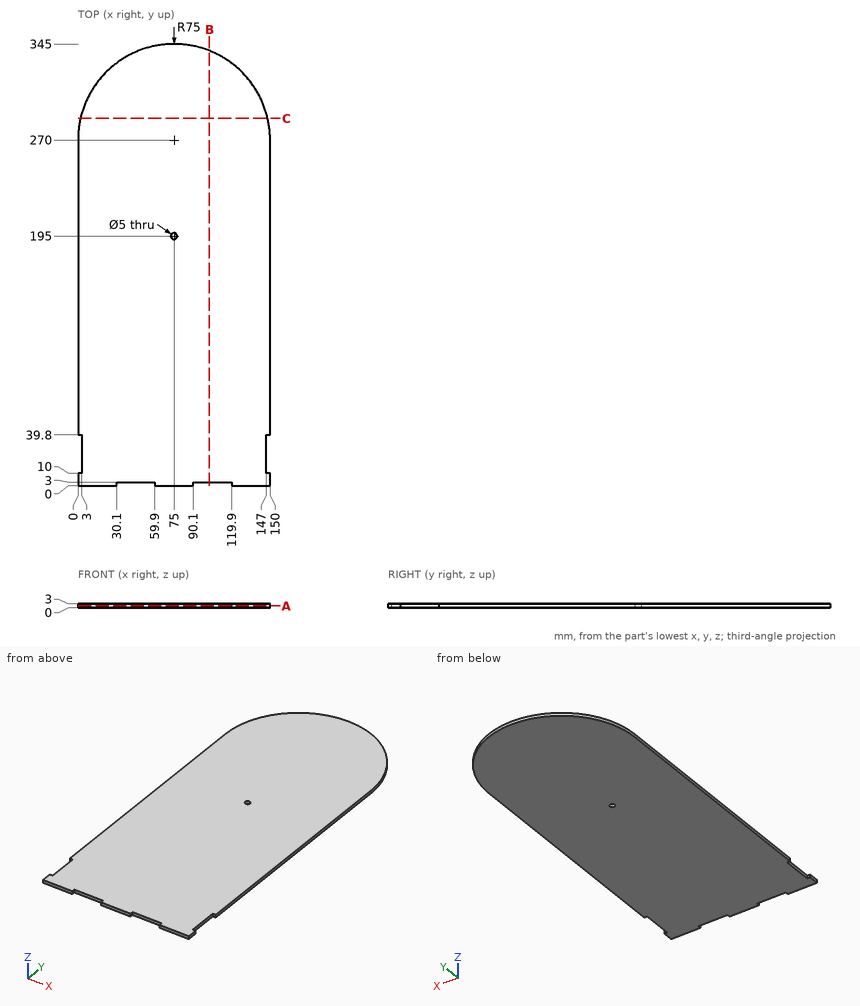
Here's the drawing with two shaded views (mm, measured from the low corner). I have some questions. Coordinates: 2 decimals unless noted, no trailing zeros. Loops run counter-clockwise (first coordinate to the right, second up) from the corner with the lowest first, then second, coordinate; pieces in that order, holes last. Notation, with made-up numbers: M -37.75,70.25 L -28.75,70.25 A13 ccw -28.75,77.25 Z; hole C 7.5,-17.75 d4. An arc over 180 degrees is marked long. Return JSON: item names as keys, results as strings. Group by question number.
Item 1: I'm going to push flat-ended pins straight in: pin 1 Ø1.5 at (y, z) = (25.5, 1) entering from +X; pin 2 Ø1.5 at (x, z) = (52, 1) entering from -Y. Where does each tip first touch, or does it pass through?
Item 2: Imagine slicing it at C-C (y = 287). Please give me the cut outline in (x, z), and give its area (3 significant figures).
Item 3: Imagine slicing it at B-B (x = 102.5). Please give me the cut outline in (y, z).
Item 4: If I drill on L1, parallel to Y at x = 75, z = 1; L2, parallel to X at y = 195, z = 1.85; L3, parallel to Y at x = 44.5, z = 2.45, over which ranges is the centre line in solid material (lowest first)? Write a range as from..to.
Item 5: Imagine slicing it at A-A (z = 1.45). Please give me the cut outline in (x, y).
Verdict:
{
 "1": {"pin 1": "stops at x = 147", "pin 2": "stops at y = 3"},
 "2": {"outline": "M 1.95,0 L 148.05,0 L 148.05,3 L 1.95,3 Z", "area": "438 mm^2"},
 "3": {"outline": "M 3,0 L 339.78,0 L 339.78,3 L 3,3 Z"},
 "4": {"L1": "y = 0..192.5, 197.5..345", "L2": "x = 0..72.5, 77.5..150", "L3": "y = 3..338.52"},
 "5": {"outline": "M 0,0 L 30.1,0 L 30.1,3 L 59.9,3 L 59.9,0 L 90.1,0 L 90.1,3 L 119.9,3 L 119.9,0 L 150,0 L 150,10 L 147,10 L 147,39.8 L 150,39.8 L 150,270 A75 ccw 0,270 L 0,39.8 L 3,39.8 L 3,10 L 0,10 Z; hole C 75,195 d5"}
}
